from build123d import *

# Parameters (mm, degrees)
SKETCH1_W           = 127.635
SKETCH1_H           = 127.635
MAIN_PLATE_DEPTH    = 12.7
SKETCH9_R           = 85.725
BOSS_EXTRUDE1_DEPTH = 12.7
SKETCH10_R          = 95.25
SKETCH10_R_2        = 85.4075
CUT_EXTRUDE1_DEPTH  = 167.64
SKETCH18_R          = 85.4075
SKETCH18_R_2        = 79.375
BOSS_EXTRUDE2_DEPTH = 38.1
SKETCH15_R          = 2.159
CUT_EXTRUDE3_DEPTH  = 88.9
CIRPATTERN1_COUNT   = 3
SKETCH23_R          = 79.375
CUT_EXTRUDE6_DEPTH  = 111.600000066


with BuildPart() as part:
    # Sketch1 → Main Plate (new body)
    with BuildSketch(Plane(origin=(0, 0, 0), x_dir=(1, 0, 0), z_dir=(0, 1, 0))):
        with Locations((63.8175, 63.8175)):
            Rectangle(SKETCH1_W, SKETCH1_H)
    extrude(amount=MAIN_PLATE_DEPTH)

    # Sketch9 → Boss-Extrude1 (add)
    with BuildSketch(Plane(origin=(0, 12.7, 0), x_dir=(1, 0, 0), z_dir=(0, 1, 0))):
        with Locations((63.8175, 63.8175)):
            Circle(SKETCH9_R)
    extrude(amount=-BOSS_EXTRUDE1_DEPTH)

    # Sketch10 → Cut-Extrude1 (cut)
    with BuildSketch(Plane(origin=(0, 12.7, 0), x_dir=(1, 0, 0), z_dir=(0, 1, 0))):
        with Locations((63.8175, 63.8175)):
            Circle(SKETCH10_R)
        with Locations((63.8175, 63.8175)):
            Circle(SKETCH10_R_2, mode=Mode.SUBTRACT)
    extrude(amount=-CUT_EXTRUDE1_DEPTH, mode=Mode.SUBTRACT)

    # Sketch18 → Boss-Extrude2 (add)
    with BuildSketch(Plane(origin=(0, 6.35, 0), x_dir=(1, 0, 0), z_dir=(0, 1, 0))):
        with Locations((63.8175, 63.8175)):
            Circle(SKETCH18_R)
        with Locations((63.8175, 63.8175)):
            Circle(SKETCH18_R_2, mode=Mode.SUBTRACT)
    extrude(amount=BOSS_EXTRUDE2_DEPTH)

    # Sketch15 → Cut-Extrude3 (cut)
    with BuildSketch(Plane(origin=(166.221610148, 0, 178.614251028), x_dir=(-0.866025404, 0, -0.5), z_dir=(0.5, 0, -0.866025404))):
        with Locations((209.900436354, 22.225)):
            Circle(SKETCH15_R)
        with Locations((209.900436354, 38.1)):
            Circle(SKETCH15_R)
    cut_extrude3 = extrude(amount=CUT_EXTRUDE3_DEPTH, mode=Mode.SUBTRACT)

    # CirPattern1: Cut-Extrude3 ×3 about axis
    cirpattern1_axis = Axis((63.8175, -154.94, -63.8175), (0, 1, 0))
    for i in range(1, CIRPATTERN1_COUNT):
        add(cut_extrude3.rotate(cirpattern1_axis, i * 360 / CIRPATTERN1_COUNT), mode=Mode.SUBTRACT)

    # Sketch23 → Cut-Extrude6 (cut)
    with BuildSketch(Plane(origin=(0, 12.7, 0), x_dir=(1, 0, 0), z_dir=(0, 1, 0))):
        with Locations((63.8175, 63.8175)):
            Circle(SKETCH23_R)
        with BuildLine():
            Line((13.678739997, 125.352005526), (7.552270878, 134.237860218))
            Line((7.552270878, 134.237860218), (-19.267108419, 125.320629884))
            Line((-19.267108419, 125.320629884), (-48.79695837, 60.397770071))
            Line((-48.79695837, 60.397770071), (-9.884344094, 7.052469015))
            Line((-9.884344094, 7.052469015), (6.959175986, -7.46308736))
            Line((6.959175986, -7.46308736), (13.678739997, 2.282994474))
            ThreePointArc((13.678739997, 2.282994474), (-15.5575, 63.8175), (13.678739997, 125.352005526))
        make_face()
        with BuildLine():
            Line((142.177324996, 76.471687114), (152.935935453, 77.334437661))
            Line((152.935935453, 77.334437661), (158.623077101, 105.019316613))
            Line((158.623077101, 105.019316613), (117.163156193, 163.054346747))
            Line((117.163156193, 163.054346747), (51.508463168, 156.027684783))
            Line((51.508463168, 156.027684783), (30.515862556, 148.698546693))
            Line((30.515862556, 148.698546693), (35.596435007, 138.00619264))
            ThreePointArc((35.596435007, 138.00619264), (103.505, 132.558266425), (142.177324996, 76.471687114))
        make_face()
        with BuildLine():
            Line((35.596435007, -10.37119264), (30.964293669, -20.119797879))
            Line((30.964293669, -20.119797879), (52.096531318, -38.887446496))
            Line((52.096531318, -38.887446496), (123.086302178, -31.999616818))
            Line((123.086302178, -31.999616818), (149.828380926, 28.372346201))
            Line((149.828380926, 28.372346201), (153.977461458, 50.217040667))
            Line((153.977461458, 50.217040667), (142.177324996, 51.163312886))
            ThreePointArc((142.177324996, 51.163312886), (103.505, -4.923266425), (35.596435007, -10.37119264))
        make_face()
    extrude(amount=CUT_EXTRUDE6_DEPTH, mode=Mode.SUBTRACT)


solid = part.part
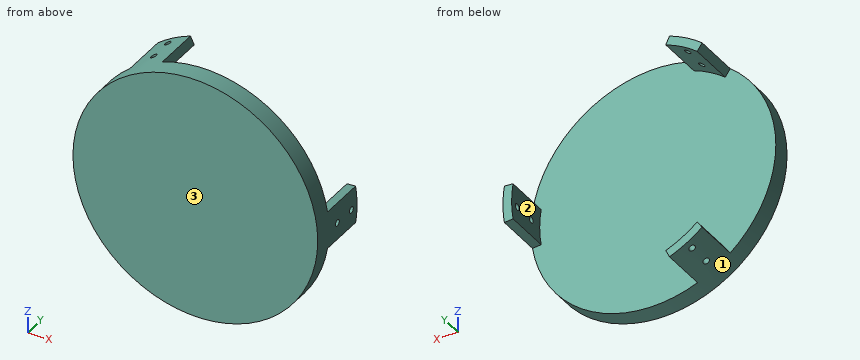
Source: CAD feature listing. Evaluate the final solid. Frame: model axes, mm. Face numbers are marked on the shaded views. Coordinates: 2 decimals unless noted, no trailing zeros. Loops run counter-clockwise (first coordinate to the right, second up) from the corner with the lowest first, then second, coordinate; pieces in that order, holes last. Notation, with made-up numbers: (76, 27.5) -> (100, 27.5) arc R6 ccw to (100, 32.5) -> close; hole circle Ø2 at (62.5, 13.25). An arc over 180 degrees is marked (long way). Answer in a Markdown table with one row per item. Add a question column.
Q1. Section C-C on z = 0.5. Return the cut outline in (x, y).
Q2. Pull-direction query (Z, two-part tool) for the marked faces 1, 2 and 3; classes: pulls with the +Z half, pulls with the -Z half, needs draft (parallel to the pull), parting line crosses it, or undercut.
Q3. Section D-D on x = 124.5. Return the cut outline in (y, z), and give its area (3 significant figures).
Q4. Section B-B on x = 29. Return the cut outline in (y, z), and give its area (3 significant figures).
Q5. Contact query for flat-ended pins moving along their axis: pin 1 Ø8 at (x, z) = (79, -4) entering from +Y; pin 2 Ø8 at (y, z) = (6, -85.5) entering from -X; pin 3 Ø6 at (x, y) = (83.5, 7.5) entering from +Z; pin 4 Ø8 at (x, z) = (-2, -59.5) entering from -Y. Output: stop coordinate, or through.
Q6. Ray query, line 1 along Y through (x, z) = (72.5, -12.5); line 2 along Z through (x, y) = (146.25, 38.1); line 3 along Z through (x, y) = (145, 38). Return the intervals inside material, ascending.
Q7. Section A-A on y = 38.1. Give the number of separate pieces and of enclosed holes in the cut face, and give its area (3 significant figures).
Computed values:
| question | item | result |
|---|---|---|
| 1 | outline | (7.62, 0) -> (120.01, 0) -> (120.01, 12.7) -> (17.3, 12.7) -> (17.3, 44.45) -> (11.76, 44.45) -> (11.76, 12.7) -> (7.62, 12.7) -> close |
| 2 | face 1 | parting line crosses it |
| 2 | face 2 | undercut |
| 2 | face 3 | needs draft |
| 3 | outline | (0, -123.92) -> (12.7, -123.92) -> (12.7, -3.72) -> (0, -3.72) -> close |
| 3 | area | 1,530 mm^2 |
| 4 | outline | (0, -141.81) -> (44.45, -141.81) -> (44.45, -135.15) -> (12.7, -135.15) -> (12.7, 7.51) -> (44.45, 7.51) -> (44.45, 14.17) -> (0, 14.17) -> close |
| 4 | area | 2,400 mm^2 |
| 5 | pin 1 | stops at y = 12.7 |
| 5 | pin 2 | stops at x = -19.74 |
| 5 | pin 3 | stops at z = 19.94 |
| 5 | pin 4 | stops at y = 0 |
| 6 | line 1 | y = 0 to 12.7 |
| 6 | line 2 | z = -76.8 to -65.98, -61.66 to -50.84 |
| 6 | line 3 | z = -76.7 to -65.97, -61.66 to -50.94 |
| 7 | separate pieces | 6 |
| 7 | enclosed holes | 0 |
| 7 | area | 391 mm^2 |
